Verification items for the finished model (mm, model axes). Face numbers are marked on the shaded views. A direction names the side the tool comes from. Round coordinates to 2 decimals unless told otherwise and drop trailing zeros. Write each loop counter-clockwise with the first axis right and the second up, starting at its lowest first coordinate (ties: lowest second). Pieces come first, ordered by that corner, then holes.
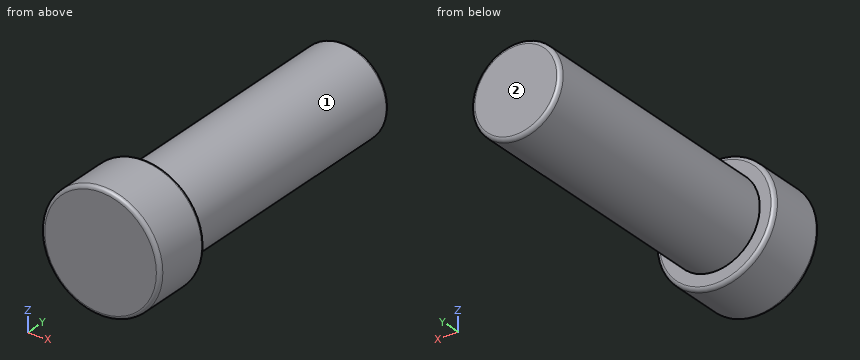
Autodesk Inventor part; units mm, degrees
ref_plane "YZ Plane" through (0, 0, 0) normal (1, 0, 0) x (0, 1, 0)
ref_plane "XZ Plane" through (0, 0, 0) normal (0, 1, 0) x (-1, 0, 0)
ref_plane "XY Plane" through (0, 0, 0) normal (0, 0, 1) x (1, 0, 0)
sketch "Sketch2" plane through (0, 0, 0) normal (0, 0, 1) x (1, 0, 0)
  line L0 (1.2, 0) -> (1.6, 0)
  line L1 (1.6, 0) -> (1.6, -1.6)
  line L2 (1.6, -1.6) -> (0, -1.6)
  line L3 (0, -1.6) -> (0, 7.2)
  line L4 (0, 7.2) -> (1.2, 7.2)
  line L5 (1.2, 7.2) -> (1.2, 0)
  point P0 (0, 0)
  dimension "d0" = 3.2
  dimension "d1" = 2.4
  dimension "d2" = 1.6
  dimension "d3" = 7.2
revolve "Revolution1" add sketch "Sketch2" angle 360 about axis through (0, -1.6, 0) along (0, 1, 0)
fillet "Fillet1" radius 0.1 3 edges at (-1.2, 7.2, 0) (-1.6, 0, 0) (-1.6, -1.6, 0)
properties part number "u9208" material "Steel"
Q1. Material ranges on line 1 along X through (y, z) = (2.25, 0.05); line 2 along Y through (x, z) = (0.45, 1.45); line 3 along X through (y, z) = (1.5, -1.05), recorded low to high.
Recorded:
line 1: x = -1.2 to 1.2
line 2: y = -1.6 to 0
line 3: x = -0.58 to 0.58
Q2. Depth check by flat-ended pin: P1, Ø1, axis at x = 1, y = 6, coming from the +Z side; P2, Ø1, axis at x = -1.5, z = -1, coming from the +Y side. Enter the tip coordinate at first touch or a pass-through.
Recorded:
P1: stops at z = 1.09
P2: stops at y = 0
Q3. Tool access check on the marked faces 1 and 2. Record the directions out of +Z, -Z, +X, -X, +Y, -Y that give a thin tool (end or side, any length) a straight path to the whole face; none if there is none.
Recorded:
face 1: +Y
face 2: +Z, -Z, +X, -X, +Y
Q4. Sectioned sample at D-D (y = 6). Enter the section's corners in (x, z), plus the area to 3 significant figures.
Recorded:
outline: circle Ø2.4 at (0, 0)
area: 4.52 mm2
Q5. Sectioned sample at A-A (x = 0). Enter the section's corners in (y, z).
Recorded:
outline: (-1.6, -1.5) arc R0.1 ccw to (-1.5, -1.6) - (-0.1, -1.6) arc R0.1 ccw to (0, -1.5) - (0, -1.2) - (7.1, -1.2) arc R0.1 ccw to (7.2, -1.1) - (7.2, 1.1) arc R0.1 ccw to (7.1, 1.2) - (0, 1.2) - (0, 1.5) arc R0.1 ccw to (-0.1, 1.6) - (-1.5, 1.6) arc R0.1 ccw to (-1.6, 1.5) - close
Q6. Sectioned sample at C-C (y = -1). Enter the section's corners in (x, z).
Recorded:
outline: circle Ø3.2 at (0, 0)
Q7. Sectioned sample at B-B (z = 0). Enter the section's corners in (x, y), plus the area to 3 significant figures.
Recorded:
outline: (-1.6, -1.5) arc R0.1 ccw to (-1.5, -1.6) - (1.5, -1.6) arc R0.1 ccw to (1.6, -1.5) - (1.6, -0.1) arc R0.1 ccw to (1.5, 0) - (1.2, 0) - (1.2, 7.1) arc R0.1 ccw to (1.1, 7.2) - (-1.1, 7.2) arc R0.1 ccw to (-1.2, 7.1) - (-1.2, 0) - (-1.5, 0) arc R0.1 ccw to (-1.6, -0.1) - close
area: 22.4 mm2
